```python
from build123d import *

# Parameters (mm, degrees)
EXTRUDE_1_DEPTH          = 750
CUT_EXTRUDE_1_DEPTH      = 770.849985387
CUT_EXTRUDE_1_DEPTH_BACK = 770.849985387
SKETCH_2_R               = 2
HOLE_WIZARD_M61_D        = 5


with BuildPart() as part:
    # Эскиз1 → Бобышка-Вытянуть1 (new, symmetric)
    with BuildSketch(Plane.XY):
        with BuildLine():
            Line((71.5, 0), (-71.5, 0))
            ThreePointArc((-71.5, 0), (-78.571067812, 2.928932188), (-81.5, 10))
            Line((-81.5, 10), (-81.5, 60))
            Line((-81.5, 60), (-76.5, 60))
            Line((-76.5, 60), (-76.5, 10))
            ThreePointArc((-76.5, 10), (-75.035533906, 6.464466094), (-71.5, 5))
            Line((-71.5, 5), (71.5, 5))
            ThreePointArc((71.5, 5), (75.035533906, 6.464466094), (76.5, 10))
            Line((76.5, 10), (76.5, 60))
            Line((76.5, 60), (81.5, 60))
            Line((81.5, 60), (81.5, 10))
            ThreePointArc((81.5, 10), (78.571067812, 2.928932188), (71.5, 0))
        make_face()
    extrude(amount=EXTRUDE_1_DEPTH, both=True)

    # Эскиз2 → Вырез-Вытянуть1 (cut, two sides: drawn at the far end of the back side and taken through both)
    with BuildSketch(Plane(origin=(81.5, 0, 0), x_dir=(0, 0, -1), z_dir=(1, 0, 0)).offset(-CUT_EXTRUDE_1_DEPTH_BACK)):
        with Locations((-600, 24.9115)):
            Circle(SKETCH_2_R)
        with Locations((-700, 24.9115)):
            Circle(SKETCH_2_R)
    extrude(amount=CUT_EXTRUDE_1_DEPTH + CUT_EXTRUDE_1_DEPTH_BACK, mode=Mode.SUBTRACT)

    # Отверстие обработанное метчиком M61 (through all)
    with Locations(Plane(origin=(81.5, 0, 0), x_dir=(0, 0, -1), z_dir=(1, 0, 0))):
        with Locations((-600, 24.9115), (-700, 24.9115)):
            Hole(HOLE_WIZARD_M61_D / 2)


solid = part.part
```
Source: CAD feature listing. Evaluate the final solid. Frame: model axes, mm. A direction names the side the tool comes from. Coordinates: 2 decimals unless noted, no trailing zeros. Loops run counter-clockwise (first coordinate to the right, second up) from the corner with the lowest first, then second, coordinate; pieces in that order, holes last. Notation, with made-up numbers: M 46,-33.75 L 53,-33.75 A13 cw 53,-15.75 Z; hole C 3,72.25 d6. An arc over 180 degrees is marked long. Use a Markdown table: item, result. Add a question column.
Q1. First-contact query: pin 1 (1.5 mm diameter, centred on x = 53.5, z = 586, fed in from +Y). Flat tip, straight axial feed; report the tip coordinate or a pass-through.
Q2. Material intervals for L1, parallel to X at y = 19, z = -291.5; L2, parallel to Y at x = -80.25, z = 700; L3, parallel to Y at x = -0.5, z = 226.5, sorted ascending.
Q3. Draft query along X for faces 1 (the flat face through (-1, 5, 10)), 2 (the flat face through (81.5, 35, 10)), 3 (the flat face through (-76.5, 35, 10)), 4 (the flat face through (1, 0, 10)). Return one class per face: pulls with the +X half, pulls with the -X half, needs draft (parallel to the pull), parting line crosses it, or undercut.
Q4. Section query B-B, the plane x = 56. Return loops of the section in (y, z), and give its area (3 significant figures).
Q5. Section query A-A, the plane z = 491. Return loops of the section in (x, y), and give its area (3 significant figures).
Q6. Access query for faces 5 (the flat face through (76.5, 35, 10)), 6 (the flat face through (-81.5, 35, 10)). Directions: +Z, -Z, +X, -X, +Y, -Y. A direction counts if a zero-diameter tool reaches every point of the face in a straight line with its end or side. Return the directions, or none.
Result:
| question | item | result |
|---|---|---|
| 1 | pin 1 | stops at y = 5 |
| 2 | L1 | x = -81.5 to -76.5, 76.5 to 81.5 |
| 2 | L2 | y = 5.16 to 22.41, 27.41 to 60 |
| 2 | L3 | y = 0 to 5 |
| 3 | face 1 | undercut |
| 3 | face 2 | pulls with the +X half |
| 3 | face 3 | undercut |
| 3 | face 4 | needs draft |
| 4 | outline | M 0,-750 L 5,-750 L 5,750 L 0,750 Z |
| 4 | area | 7,500 mm2 |
| 5 | outline | M -81.5,10 A10 ccw -71.5,0 L 71.5,0 A10 ccw 81.5,10 L 81.5,60 L 76.5,60 L 76.5,10 A5 cw 71.5,5 L -71.5,5 A5 cw -76.5,10 L -76.5,60 L -81.5,60 Z |
| 5 | area | 1,330 mm2 |
| 6 | face 5 | +Z, -Z, +Y |
| 6 | face 6 | +Z, -Z, -X, +Y, -Y |
